from build123d import *

# Parameters (mm, degrees)
SKETCH_1_W             = 150
SKETCH_1_H             = 80
SKETCH_1_R             = 1.3
SKETCH_1_R_2           = 22
EXTRUDE_1_DEPTH        = 5
SKETCH_2_R             = 2.34
CUT_EXTRUDE_1_DEPTH    = 2.5
SKETCH_3_R             = 1.55
SKETCH_3_R_2           = 1.582849294
CUT_EXTRUDE_3_DEPTH    = 12.5
CUT_EXTRUDE_5_DEPTH    = 8
FILLET_3_R             = 2
FILLET_3_OF_MIRROR_2_R = 2
EXTRUDE_4_DEPTH        = 5
FILLET_5_R             = 5
SKETCH_11_R            = 1.55
CUT_EXTRUDE_7_DEPTH    = 25
SKETCH_12_R            = 2.05
CUT_EXTRUDE_8_DEPTH    = 10
CUT_EXTRUDE_9_DEPTH    = 10
FILLET_6_R             = 1
EXTRUDE_5_DEPTH        = 5


with BuildPart() as part:
    # 草图1 → 凸台-拉伸1 (new body)
    with BuildSketch(Plane.XY):
        with Locations((-5, 0)):
            Rectangle(SKETCH_1_W, SKETCH_1_H)
        with Locations((0, -24.5)):
            Circle(SKETCH_1_R, mode=Mode.SUBTRACT)
        with Locations((-21.217622393, -12.25)):
            Circle(SKETCH_1_R, mode=Mode.SUBTRACT)
        with Locations((-21.217622393, 12.25)):
            Circle(SKETCH_1_R, mode=Mode.SUBTRACT)
        Circle(SKETCH_1_R_2, mode=Mode.SUBTRACT)
        with Locations((0, 24.5)):
            Circle(SKETCH_1_R, mode=Mode.SUBTRACT)
        with Locations((21.217622393, 12.25)):
            Circle(SKETCH_1_R, mode=Mode.SUBTRACT)
        with Locations((21.217622393, -12.25)):
            Circle(SKETCH_1_R, mode=Mode.SUBTRACT)
    extrude(amount=EXTRUDE_1_DEPTH)

    # 草图2 → 切除-拉伸1 (cut)
    with BuildSketch(Plane.XY.offset(5)):
        with Locations((-21.217622393, 12.25)):
            Circle(SKETCH_2_R)
        with Locations((0, 24.5)):
            Circle(SKETCH_2_R)
        with Locations((21.217622393, 12.25)):
            Circle(SKETCH_2_R)
        with Locations((21.217622393, -12.25)):
            Circle(SKETCH_2_R)
        with Locations((0, -24.5)):
            Circle(SKETCH_2_R)
        with Locations((-21.217622393, -12.25)):
            Circle(SKETCH_2_R)
    extrude(amount=-CUT_EXTRUDE_1_DEPTH, mode=Mode.SUBTRACT)

    # 草图3 → 切除-拉伸3 (cut)
    with BuildSketch(Plane.XY.offset(5)):
        with Locations((-60, -25)):
            Circle(SKETCH_3_R)
        with Locations((-60, -5)):
            Circle(SKETCH_3_R_2)
        with Locations((-60, 25)):
            Circle(SKETCH_3_R)
        with Locations((-60, 5)):
            Circle(SKETCH_3_R_2)
    extrude(amount=-CUT_EXTRUDE_3_DEPTH, mode=Mode.SUBTRACT)

    # 草图4 → 切除-拉伸5 (cut)
    with BuildSketch(Plane.XY.offset(5)):
        Polygon((-58, 35), (-30, 35), (-58, 11.505210327), align=None)
        Polygon((-35, 25.582872687), (-58, 6.28358117), (-35, 6.28358117), align=None)
    cut_extrude_5 = extrude(amount=-CUT_EXTRUDE_5_DEPTH, mode=Mode.SUBTRACT)

    # 圆角3
    fillet_3_edges = [part.edges().sort_by_distance(p)[0] for p in [
        (-35, 6.28358117, 2.5),
        (-58, 6.28358117, 2.5),
        (-35, 25.582872687, 2.5),
        (-30, 35, 2.5),
        (-58, 11.505210327, 2.5),
        (-58, 35, 2.5),
    ]]
    fillet(fillet_3_edges, radius=FILLET_3_R)

    # 镜向2: 切除-拉伸5 across plane
    add(cut_extrude_5.mirror(Plane.ZX), mode=Mode.SUBTRACT)

    # 圆角3 of 镜向2
    fillet_3_of_mirror_2_edges = [part.edges().sort_by_distance(p)[0] for p in [
        (-35, -6.28358117, 2.5),
        (-58, -6.28358117, 2.5),
        (-35, -25.582872687, 2.5),
        (-30, -35, 2.5),
        (-58, -11.505210327, 2.5),
        (-58, -35, 2.5),
    ]]
    fillet(fillet_3_of_mirror_2_edges, radius=FILLET_3_OF_MIRROR_2_R)

    # 草图10 → 凸台-拉伸4 (add)
    with BuildSketch(Plane.XY.offset(5)):
        Polygon((-80, -40), (-127.053079228, -7.053079228), (-80, 40), align=None)
    extrude(amount=-EXTRUDE_4_DEPTH)

    # 圆角5
    fillet_5_edges = [part.edges().sort_by_distance(p)[0] for p in [
        (-127.053079228, -7.053079228, 2.5),
    ]]
    fillet(fillet_5_edges, radius=FILLET_5_R)

    # 草图11 → 切除-拉伸7 (cut)
    with BuildSketch(Plane.XY.offset(5)):
        with Locations((-15.75, 27.279800219)):
            Circle(SKETCH_11_R)
        with Locations((15.75, 27.279800219)):
            Circle(SKETCH_11_R)
        with Locations((31.5, 0)):
            Circle(SKETCH_11_R)
        with Locations((15.75, -27.279800219)):
            Circle(SKETCH_11_R)
        with Locations((-15.75, -27.279800219)):
            Circle(SKETCH_11_R)
        with Locations((-31.5, 0)):
            Circle(SKETCH_11_R)
    extrude(amount=-CUT_EXTRUDE_7_DEPTH, mode=Mode.SUBTRACT)

    # 草图12 → 切除-拉伸8 (cut)
    with BuildSketch(Plane.XY.offset(5)):
        with Locations((35, 25)):
            Circle(SKETCH_12_R)
        with Locations((65, 25)):
            Circle(SKETCH_12_R)
        with Locations((65, -25)):
            Circle(SKETCH_12_R)
        with Locations((35, -25)):
            Circle(SKETCH_12_R)
    extrude(amount=-CUT_EXTRUDE_8_DEPTH, mode=Mode.SUBTRACT)

    # 草图13 → 切除-拉伸9 (cut)
    with BuildSketch(Plane.XY.offset(5)):
        Polygon((35, 19), (35, -19), (46.4, 0), align=None)
        Polygon((65, -19), (53.6, 0), (65, 19), align=None)
        Polygon((41, 19), (50, 4), (59, 19), align=None)
        Polygon((50, -4), (59, -19), (41, -19), align=None)
    extrude(amount=-CUT_EXTRUDE_9_DEPTH, mode=Mode.SUBTRACT)

    # 圆角6
    fillet_6_edges = [part.edges().sort_by_distance(p)[0] for p in [
        (41, 19, 2.5),
        (59, 19, 2.5),
        (50, 4, 2.5),
        (65, 19, 2.5),
        (65, -19, 2.5),
        (53.6, 0, 2.5),
        (41, -19, 2.5),
        (50, -4, 2.5),
        (59, -19, 2.5),
        (35, 19, 2.5),
        (46.4, 0, 2.5),
        (35, -19, 2.5),
    ]]
    fillet(fillet_6_edges, radius=FILLET_6_R)

    # 草图14 → 凸台-拉伸5 (add)
    with BuildSketch(Plane.XY.offset(5)):
        Polygon((-80, -40), (-65.718519933, -50), (70, -50), (70, -40), align=None)
    extrude(amount=-EXTRUDE_5_DEPTH)


solid = part.part
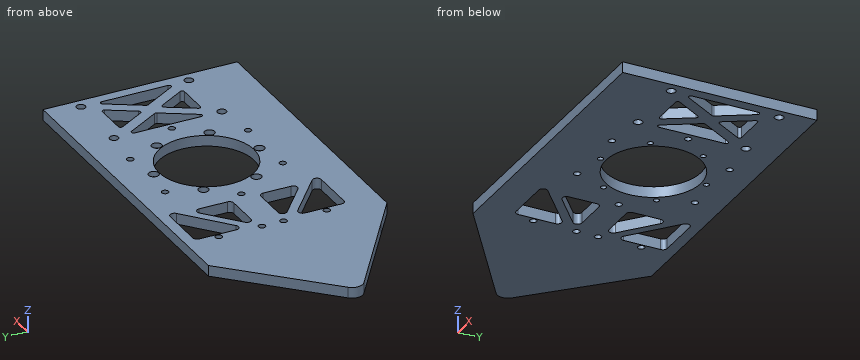
Here's how the part is built. I have some questions about the finished solid (model axes, mm). Give positions to 0.01 mm unless a question says otherwise; leave off trailing zeros. Answer as a JSON object with one key per item and string values. Group by question number.
1) Suppose I cut it at A-A, the plane z = 3.6. Count the separate pieces of the cut face and the enclosed holes in it, plus the area to 3 significant figures.
2) I'm going to push flat-ended pins straight in: pin 1 Ø3 at (x, y) = (0, 24.5) entering from +Z; pin 2 Ø4 at (x, y) = (-21.22, -12.25) entering from -Z; pin 3 Ø1.5 at (y, z) = (-14, 3) entering from -X. Where does each tip first touch, or does it pass through?
3) Please list where these lines run through material, in increasing order: L1, parallel to Y at x = -60, z = 3.65; L2, parallel to Y at x = -15.75, z = 2.3; L3, parallel to X at y = -17.5, z = 3.45. Write a range as [from, to].
Results found:
{
 "1": {"separate pieces": "1", "enclosed holes": "29", "area": "11,800 mm²"},
 "2": {"pin 1": "z = 2.5", "pin 2": "z = 0", "pin 3": "x = -118.2"},
 "3": {"L1": "[-50, -26.55], [-23.45, -6.58], [-3.42, 3.42], [6.58, 23.45], [26.55, 40]", "L2": "[-50, -28.83], [-25.73, -15.36], [15.36, 25.73], [28.83, 40]", "L3": "[-112.13, -58], [-50.86, -44.63], [-35, -13.33], [13.33, 41.9], [58.1, 70]"}
}
